```python
from build123d import *

# Parameters (mm, degrees)
SKETCH1_R                 = 78.359
BOSS_EXTRUDE1_DEPTH       = 25.4
SKETCH6_R                 = 76.1746
BOSS_EXTRUDE5_DEPTH       = 9.525
SKETCH7_R                 = 76.1746
BOSS_EXTRUDE6_DEPTH       = 9.525
SKETCH8_R                 = 73.025
CUT_EXTRUDE5_DEPTH        = 34.925
SKETCH3_R                 = 2
CUT_EXTRUDE2_DEPTH        = 9.525
CUT_EXTRUDE3_START        = 25.4
SKETCH1_7_R               = 78.359
SKETCH1_7_R_2             = 76.1746
CUT_EXTRUDE3_DEPTH        = 9.525
CIRPATTERN2_COUNT         = 3
SKETCH4_R                 = 73.025
BOSS_EXTRUDE4_DEPTH       = 9.525
CIRPATTERN3_COUNT         = 4
SKETCH9_R                 = 3.3
CUT_EXTRUDE6_DEPTH        = 45.4500001
SKETCH10_R                = 82.322787435
CUT_EXTRUDE7_DEPTH        = 35.9250001
TAP_DRILL_FOR_4_40_TAP1_D = 2.2606
CUT_EXTRUDE9_DEPTH        = 10.5250001


with BuildPart() as part:
    # Sketch1 → Boss-Extrude1 (new body)
    with BuildSketch(Plane(origin=(0, 0, 0), x_dir=(1, 0, 0), z_dir=(0, 1, 0))):
        Circle(SKETCH1_R)
    extrude(amount=BOSS_EXTRUDE1_DEPTH)

    # Sketch6 → Boss-Extrude5 (add)
    with BuildSketch(Plane(origin=(0, 25.4, 0), x_dir=(1, 0, 0), z_dir=(0, 1, 0))):
        Circle(SKETCH6_R)
    extrude(amount=BOSS_EXTRUDE5_DEPTH)

    # Sketch7 → Boss-Extrude6 (add)
    with BuildSketch(Plane.XZ):
        Circle(SKETCH7_R)
    extrude(amount=BOSS_EXTRUDE6_DEPTH)

    # Sketch8 → Cut-Extrude5 (cut)
    with BuildSketch(Plane.XZ.offset(9.525)):
        Circle(SKETCH8_R)
    extrude(amount=-CUT_EXTRUDE5_DEPTH, mode=Mode.SUBTRACT)

    # Sketch3 → Cut-Extrude2 (cut)
    with BuildSketch(Plane(origin=(0, 0, -76.1746), x_dir=(-1, 0, 0), z_dir=(0, 0, -1))):
        with Locations((0, 30.1625)):
            Circle(SKETCH3_R)
        with Locations((0, -4.7625)):
            Circle(SKETCH3_R)
    cut_extrude2 = extrude(amount=-CUT_EXTRUDE2_DEPTH, mode=Mode.SUBTRACT)

    # Sketch1<7> → Cut-Extrude3 (cut)
    with BuildSketch(Plane(origin=(0, 0, 0), x_dir=(1, 0, 0), z_dir=(0, 1, 0)).offset(CUT_EXTRUDE3_START)):
        Circle(SKETCH1_7_R)
        Circle(SKETCH1_7_R_2, mode=Mode.SUBTRACT)
    cut_extrude3 = extrude(amount=-CUT_EXTRUDE3_DEPTH, mode=Mode.SUBTRACT)

    # CirPattern2: Cut-Extrude3 ×3 about axis
    cirpattern2_axis = Axis((0, 0, 0), (0, 1, 0))
    for i in range(1, CIRPATTERN2_COUNT):
        add(cut_extrude3.rotate(cirpattern2_axis, i * 360 / CIRPATTERN2_COUNT), mode=Mode.SUBTRACT)

    # Sketch4 → Boss-Extrude4 (add)
    with BuildSketch(Plane(origin=(0, 34.925, 0), x_dir=(1, 0, 0), z_dir=(0, 1, 0))):
        Circle(SKETCH4_R)
    extrude(amount=-BOSS_EXTRUDE4_DEPTH)

    # CirPattern3: Cut-Extrude2 ×4 about axis
    cirpattern3_axis = Axis((0, 0, 0), (0, 1, 0))
    for i in range(1, CIRPATTERN3_COUNT):
        add(cut_extrude2.rotate(cirpattern3_axis, i * 360 / CIRPATTERN3_COUNT), mode=Mode.SUBTRACT)

    # Sketch9 → Cut-Extrude6 (cut, through all)
    with BuildSketch(Plane(origin=(0, 34.925, 0), x_dir=(1, 0, 0), z_dir=(0, 1, 0))):
        Circle(SKETCH9_R)
        with Locations((-19.546451191, -53.703433278)):
            Circle(SKETCH9_R)
        with Locations((-36.735311894, 43.779439924)):
            Circle(SKETCH9_R)
        with Locations((56.281763085, 9.923993354)):
            Circle(SKETCH9_R)
        with Locations((18.367655947, -21.889719962)):
            Circle(SKETCH9_R)
    extrude(amount=-CUT_EXTRUDE6_DEPTH, mode=Mode.SUBTRACT)

    # Sketch10 → Cut-Extrude7 (cut, through all)
    with BuildSketch(Plane(origin=(0, 25.4, 0), x_dir=(1, 0, 0), z_dir=(0, 1, 0))):
        Circle(SKETCH10_R)
    extrude(amount=-CUT_EXTRUDE7_DEPTH, mode=Mode.SUBTRACT)

    # Tap Drill for #4-40 Tap1 (through all)
    with Locations(Plane(origin=(0, 34.925, 0), x_dir=(1, 0, 0), z_dir=(0, 1, 0))):
        with Locations((7.384214894, 20.287963683), (15.934718491, 43.780279238)):
            Hole(TAP_DRILL_FOR_4_40_TAP1_D / 2)

    # Sketch14 → Cut-Extrude9 (cut, through all)
    with BuildSketch(Plane(origin=(0, 34.925, 0), x_dir=(1, 0, 0), z_dir=(0, 1, 0))):
        with BuildLine():
            Line((14.64382936, 22.781402035), (19.893154532, 37.203804415))
            ThreePointArc((19.893154532, 37.203804415), (19.808357055, 39.145985964), (18.37506644, 40.459354836))
            Line((18.37506644, 40.459354836), (11.930654446, 42.804928978))
            ThreePointArc((11.930654446, 42.804928978), (9.988472897, 42.720131501), (8.675104025, 41.286840886))
            Line((8.675104025, 41.286840886), (3.425778853, 26.864438506))
            ThreePointArc((3.425778853, 26.864438506), (3.51057633, 24.922256957), (4.943866945, 23.608888085))
            Line((4.943866945, 23.608888085), (11.388278939, 21.263313942))
            ThreePointArc((11.388278939, 21.263313942), (13.330460488, 21.34811142), (14.64382936, 22.781402035))
        make_face()
    extrude(amount=-CUT_EXTRUDE9_DEPTH, mode=Mode.SUBTRACT)


solid = part.part
```
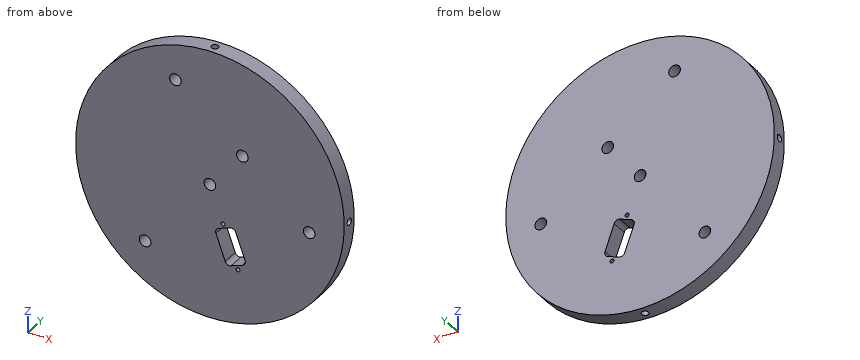
Verification items for the finished model (mm, model axes). Give positions to 0.01 mm unless a question says otherwise; leave off trailing zeros. Order: outer loops, then holes, each group sorted by start corner. A loop starts at its lowest first (then second) coordinate and runs counter-clockwise, first axis right, second up. Notation, with made-up numbers: M 10,-23.5 L 22,-23.5 A17 ccw 22,-13.5 Z; hole C 23,54.25 d2. An arc over 180 degrees is marked long. Return JSON: item names as keys, results as strings. Group by question number.
1) Section check D-D on z = -66. Record the cut outline in (x, y) (3 decimals).
2) Scan lines: line 1 (Y direction, x = -70, z = 0) (1 decimal); line 2 (X direction, y = 28.25, z = -27); line 3 (X direction, y = 30.75, z = -24.5). Record each from-to range of solid material in increasing order.
3) Section check C-C on x = -20.5. Record the cut outline in (y, z) (3 decimals), and give its area (3 significant figures).
4) Section check B-B on x = 0. Record the cut outline in (y, z) (1 decimal).
5) Go/stop test with flat-tipped pins: pin 1 Ø5.5 at (x, z) = (18.37, 21.89) entering from -Y; pin 2 Ø2 at (y, z) = (33.5, 38.5) entering from -X; pin 3 Ø3 at (y, z) = (30, -1) entering from +X; pin 4 Ø3 at (x, y) = (34.5, 31.5) entering from +Z. Record where each tip stops, or that it passes through.
6) Section check A-A on z = 0. Record the cut outline in (x, y) (1 decimal).
Answer block:
{
 "1": {"outline": "M -38.034,25.4 L 38.034,25.4 L 38.034,34.925 L -38.034,34.925 Z"},
 "2": {"line 1": "y = 25.4 to 28.2, 32.2 to 34.9", "line 2": "x = -71.23 to 3.48, 16.18 to 71.23", "line 3": "x = -72.13 to 3.76, 15.27 to 72.13"},
 "3": {"outline": "M 25.4,-73.364 L 34.925,-73.364 L 34.925,50.544 L 25.4,50.544 Z; M 25.4,56.863 L 34.925,56.863 L 34.925,73.364 L 25.4,73.364 Z", "area": "1,340 mm^2"},
 "4": {"outline": "M 25.4,-76.2 L 28.2,-76.2 L 28.2,-73 L 32.2,-73 L 32.2,-76.2 L 34.9,-76.2 L 34.9,-3.3 L 25.4,-3.3 Z; M 25.4,3.3 L 34.9,3.3 L 34.9,76.2 L 32.2,76.2 L 32.2,66.6 L 28.2,66.6 L 28.2,76.2 L 25.4,76.2 Z"},
 "5": {"pin 1": "passes through", "pin 2": "stops at x = -66.3", "pin 3": "stops at x = 76.17", "pin 4": "stops at z = 68.66"},
 "6": {"outline": "M -76.2,25.4 L -3.3,25.4 L -3.3,34.9 L -76.2,34.9 L -76.2,32.2 L -66.6,32.2 L -66.6,28.2 L -76.2,28.2 Z; M 3.3,25.4 L 76.2,25.4 L 76.2,28.2 L 66.6,28.2 L 66.6,32.2 L 76.2,32.2 L 76.2,34.9 L 3.3,34.9 Z"}
}
